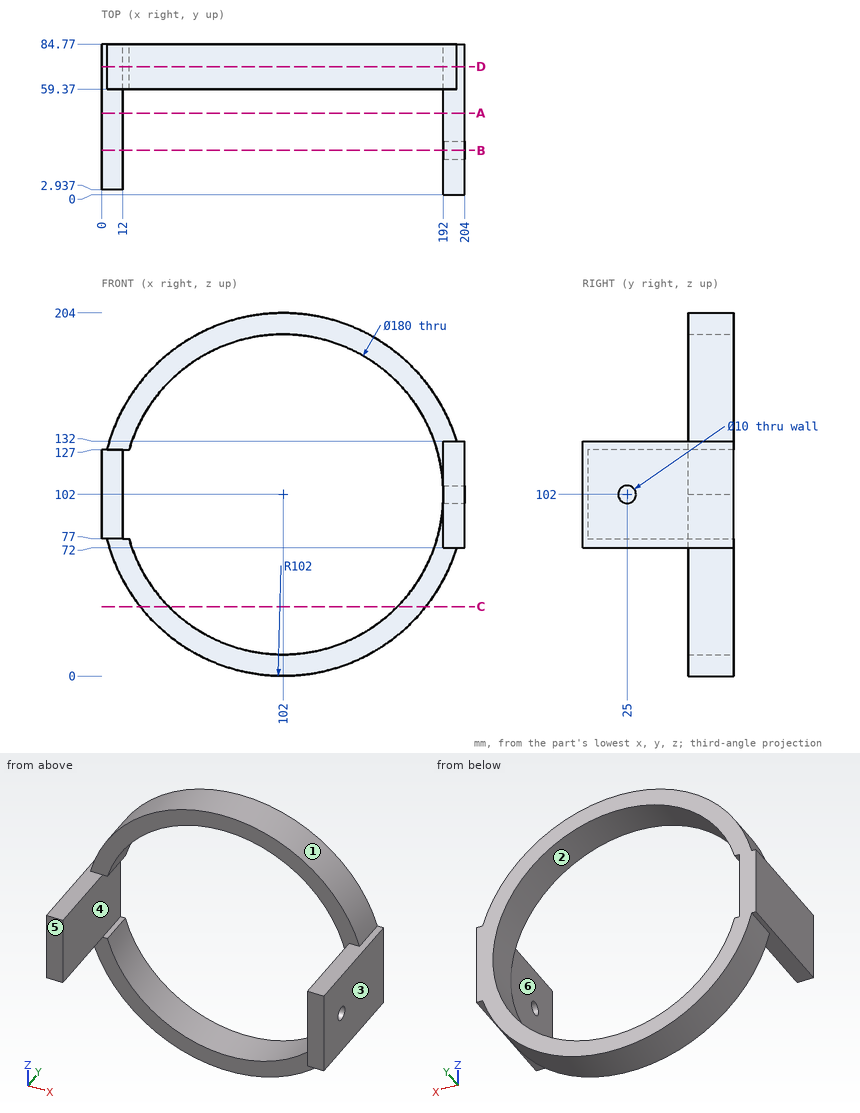
Job drawing, mm, ordinate dimensions from the low corner. One solid piece. A direction names the side the tool comes from. Give positions to 0.01 mm unless a question says otherwise; leave off trailing zeros. Loops run counter-clockwise (first coordinate to the right, second up) from the corner with the lowest first, then second, coordinate; pieces in that order, holes last. Notation, with made-up numbers: (-33.75, 39.5) -> (22.25, 39.5) arc R24 cw to (22.25, 60.5) -> close; hole circle Ø7 at (4.5, -19). An arc over 180 degrees is marked (long way). Write each question's results on one line, items separated by ' | '.
(1) Pull direction X, two halves, no side cores. Call the marked faces 1, 2 and 3: released by +X, released by -X, zero draft, split by the parting line, or undercut.
Geometry results:
face 1: split by the parting line | face 2: undercut | face 3: released by +X
(2) Cut at C-C on z = 39. List the corners of the cut face in (x, y), and give its area (3 significant figures).
Geometry results:
outline: (21.78, 59.37) -> (37.73, 59.37) -> (37.73, 84.77) -> (21.78, 84.77) -> close; (166.27, 59.37) -> (182.22, 59.37) -> (182.22, 84.77) -> (166.27, 84.77) -> close | area: 810 mm²
(3) Tool access for the marked faces 4, 5 and 6: list every direction of +Z, -Z, +X, -X, +Y, -Y with a clear straight run to the whole face (end or side of a thin tool).
Geometry results:
face 4: +Y, -Y | face 5: +Z, -Z, -X, -Y | face 6: +Z, -Z, -Y
(4) Flat gauge pins, fed straight in: pin 1 Ø4 at (x, y) = (100, 58) entering from +Z; pin 2 Ø13 at (x, z) = (7, 112) entering from -Y; pin 3 Ø4 at (x, y) = (14.5, 76) entering from -Z; pin 4 Ø10 at (x, z) = (36.5, 55) entering from +Y. Where does each tip first touch, or does it go through?
Geometry results:
pin 1: stops at z = 204 | pin 2: stops at y = 2.94 | pin 3: stops at z = 46.38 | pin 4: passes through
(5) Probe line 1 along X through (y, z) = (48, 82.5); line 2 along Y through (x, z) = (200.25, 102). List the from-to ranges inside material, lowest first.
Geometry results:
line 1: x = 0 to 12, 192 to 204 | line 2: y = 0 to 20, 30 to 84.77
(6) Cut at D-D on y = 72. List the corners of the cut face in (x, z), and give its area (3 significant figures).
Geometry results:
outline: (0, 77) -> (3.11, 77) arc R102 ccw to (199.49, 72) -> (204, 72) -> (204, 132) -> (199.49, 132) arc R102 ccw to (3.11, 127) -> (0, 127) -> close; hole (12, 77) -> (15.54, 77) arc R90 ccw (long way) to (15.54, 127) -> (12, 127) -> close | area: 7,320 mm²
(7) Cut at B-B on y = 25. List the corners of the cut face in (x, z).
Geometry results:
outline: (0, 77) -> (12, 77) -> (12, 127) -> (0, 127) -> close; (192, 72) -> (204, 72) -> (204, 97) -> (192, 97) -> close; (192, 107) -> (204, 107) -> (204, 132) -> (192, 132) -> close
(8) Cut at A-A on y = 46. List the corners of the cut face in (x, z).
Geometry results:
outline: (0, 77) -> (12, 77) -> (12, 127) -> (0, 127) -> close; (192, 72) -> (204, 72) -> (204, 132) -> (192, 132) -> close
